```python
from build123d import *

# Parameters (mm, degrees)
F0_R          = 6.3
F0_R_2        = 3.8
F1_DEPTH      = 25
F2_R          = 8.3
F2_R_2        = 6.3
F3_DEPTH      = 7.3
F3_DEPTH_BACK = 2
F4_SIZE       = 1.99999
F5_R          = 0.5


# Not quite as in the source:
# - a fillet or chamfer is up to 0.001 mm smaller than in the source, because OpenCascade refuses the exact size


with BuildPart() as f1:
    # F0 (on Top) → F1 (new body)
    with BuildSketch(Plane.XY):
        Circle(F0_R)
        Circle(F0_R_2, mode=Mode.SUBTRACT)
    extrude(amount=F1_DEPTH)

    # F2 (on face) → F3 (join, two sides)
    with BuildSketch(Plane(origin=(0, 0, 0), x_dir=(1, 0, 0), z_dir=(0, 0, -1))) as f3_sk:
        Circle(F2_R)
        Circle(F2_R_2, mode=Mode.SUBTRACT)
    extrude(amount=F3_DEPTH)
    extrude(f3_sk.sketch, amount=-F3_DEPTH_BACK)

    # F4 (size 2 in the source; OpenCascade refuses exactly that, so slightly less here)
    f4_edges = [f1.edges().sort_by_distance(p)[0] for p in [
        (-6.3, 0, 2),
    ]]
    chamfer(f4_edges, length=F4_SIZE)

    # F5
    f5_edges = [f1.edges().sort_by_distance(p)[0] for p in [
        (-3.8, 0, 25),
        (-6.3, 0, -7.3),
    ]]
    fillet(f5_edges, radius=F5_R)


solid = f1.part
```
Geometry check sheet. Reference: the model listing, model coordinates, mm. A direction names the side the tool comes from. Coordinates: 2 decimals unless noted, no trailing zeros. Write each loop counter-clockwise with the first axis right and the second up, starting at its lowest first coordinate (ties: lowest second). Pieces come first, ordered by that corner, then holes. Notation, with made-up numbers: (-22.5, 18.25) -> (-9.5, 18.25) arc R14 cw to (-9.5, 26.25) -> close; hole circle Ø8 at (7, -4.5). An arc over 180 degrees is marked (long way). Use CSV: the item, a comma, the result in double quotes. Start each with the question number.
Item 1: Depth check by flat-ended pin: pin 1 Ø1.5 at (y, z) = (-5, 21) entering from +X; pin 2 Ø1 at (x, z) = (-5.5, 4) entering from -Y; pin 3 Ø5 at (y, z) = (4, 20.5) entering from +X. Enter the tip coordinate at first touch or a pass-through.
Item 2: Cross-section at C-C, the plane z = 9.5. Record the cut outline in (x, y).
Item 3: Set-up check for faces 4 (the cylindrical face through (-5, -3.83, 14.35)), 5 (the flat face through (3, -3, 0)), 6 (the flat face through (-7, 0, -7.3)): record each of +Z, -Z, +X, -X, +Y, -Y from which the full face is reachable in a straight line by a thin tool's end or side.
Item 4: Mould release check, pull along Y, two halves, no side actions. Record for faces 1 (the flat face through (3, -4, 25)), 2 (the conical face through (6.128, -1.93, 3.875)), 3 (the cylindrical face through (-3.796, 0.167, 12.078)): released by +Y, released by -Y, zero draft, split by the parting line, or undercut.
Item 5: Thickness scan on line 1 (X direction, y = 0, z = -1.5); line 2 (Y direction, x = 0, z = 17.5). Record the ranges inside material, lowest first.
Answers:
1,pin 1,"x = 4.65"
1,pin 2,"y = -4.23"
1,pin 3,"x = 6.12"
2,outline,"circle Ø12.6 at (0, 0); hole circle Ø7.6 at (0, 0)"
3,face 4,"+Z"
3,face 5,"-Z"
3,face 6,"-Z, +X, -X, +Y, -Y"
4,face 1,"zero draft"
4,face 2,"split by the parting line"
4,face 3,"undercut"
5,line 1,"-8.3 to -6.3, 6.3 to 8.3"
5,line 2,"-6.3 to -3.8, 3.8 to 6.3"
